Model file for the job. Use its own axes, mm. Face numbers are marked on the shaded views. A direction names the side the tool comes from. Give positions to 0.01 mm unless a question says otherwise; leave off trailing zeros. Write each loop counter-clockwise with the first axis right and the second up, starting at its lowest first coordinate (ties: lowest second). Pieces come first, ordered by that corner, then holes. Notation, with made-up numbers: (60.25, -6) - (105.25, -6) arc R18 ccw to (105.25, 2) - close; hole circle Ø2 at (-24.5, 42). An arc over 180 degrees is marked (long way). One line per item, written item: value. Start each with the question number.
(1) Mould opens along Z. For the marked faces 1, 2 and 3 say: pulls with the +Z half, pulls with the -Z half, needs draft (parallel to the pull), parting line crosses it, or undercut.
(2) Cut at A-A, the plane y = 0. List the corners of the cut face in (x, z).
(3) 3-axis set-ups, long thin cutter, end or side, ignore diameter. For the marked faces 4, 5, 6 and 7: which of +Z, -Z, +X, -X, +Y, -Y reach the whole face in a straight line?
(4) Drop flat-ended pins along their axis: P1, Ø3, axis at y = 14, z = 39.5, coming from the -X side; P2, Ø3, axis at x = 13.5, z = -13, coming from the +Y side; P3, Ø17, axis at x = 0, y = 0, coming from the +Z side; P4, Ø12, axis at x = 0, y = 0, coming from the -Z side. Give the stop position or say it passes through.
(5) Cut at D-D, the plane y = 17. List the corners of the cut face in (x, z).
(6) Cut at C-C, the plane z = 19.5. List the corners of the cut face in (x, y).
(7) Probe L1, parallel to X at y = 0, z = -16; L2, parallel to Y at x = 0, z = 22.5; L3, parallel to Y at x = 0, z = 35.5. List the from-to ranges inside material, lowest first.
(8) Cut at B-B, the plane x = 0. List the corners of the cut face in (y, z).
from build123d import *

# Parameters (mm, degrees)
F0_W          = 60
F0_H          = 50
F1_DEPTH      = 25
F1_DEPTH_BACK = 25
F4_R          = 7.5
F5_DEPTH      = 75.001
F6_R          = 12.5
F7_DEPTH      = 35
F7_DEPTH_BACK = 35


with BuildPart() as f1:
    # F0 (on Top) → F1 (new body, two sides)
    with BuildSketch(Plane.XY) as f1_sk:
        Rectangle(F0_W, F0_H)
    extrude(amount=F1_DEPTH)
    extrude(f1_sk.sketch, amount=-F1_DEPTH_BACK)

    # F2 (on Front) → F3 (revolve)
    with BuildSketch(Plane.XZ):
        Polygon((-15, 40), (-15, 25), (0, 25), (0, 50), (-25, 50), (-25, 40), align=None)
    revolve(axis=Axis((0, 0, 37.5), (0, 0, -1)))

    # F4 (on face) → F5 (cut, through all)
    with BuildSketch(Plane.XY.offset(50)):
        Circle(F4_R)
    extrude(amount=-F5_DEPTH, mode=Mode.SUBTRACT)

    # F6 (on Front) → F7 (join, two sides)
    with BuildSketch(Plane.XZ) as f7_sk:
        Circle(F6_R)
    extrude(amount=F7_DEPTH)
    extrude(f7_sk.sketch, amount=-F7_DEPTH_BACK)


solid = f1.part
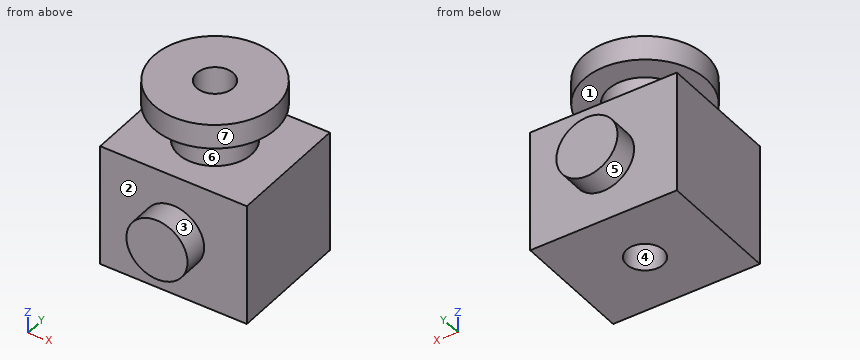
Answers follow:
1. face 1: undercut
1. face 2: needs draft
1. face 3: parting line crosses it
2. outline: (-30, -25) - (-7.5, -25) - (-7.5, -10) arc R12.5 ccw to (7.5, -10) - (7.5, -25) - (30, -25) - (30, 25) - (15, 25) - (15, 40) - (25, 40) - (25, 50) - (7.5, 50) - (7.5, 10) arc R12.5 ccw to (-7.5, 10) - (-7.5, 50) - (-25, 50) - (-25, 40) - (-15, 40) - (-15, 25) - (-30, 25) - close
3. face 4: -Z
3. face 5: +Y
3. face 6: none
3. face 7: +Z
4. P1: stops at x = -21.6
4. P2: stops at y = 25
4. P3: stops at z = 50
4. P4: stops at z = -12.5
5. outline: (-30, -25) - (30, -25) - (30, 25) - (-30, 25) - close; (-18.33, 40) - (18.33, 40) - (18.33, 50) - (-18.33, 50) - close
6. outline: (-30, -25) - (30, -25) - (30, 25) - (-30, 25) - close; hole circle Ø15 at (0, 0)
7. L1: x = -30 to -7.5, 7.5 to 30
7. L2: y = -25 to -7.5, 7.5 to 25
7. L3: y = -15 to -7.5, 7.5 to 15
8. outline: (-35, -12.5) - (-25, -12.5) - (-25, -25) - (-7.5, -25) - (-7.5, -12.5) - (7.5, -12.5) - (7.5, -25) - (25, -25) - (25, -12.5) - (35, -12.5) - (35, 12.5) - (25, 12.5) - (25, 25) - (15, 25) - (15, 40) - (25, 40) - (25, 50) - (7.5, 50) - (7.5, 12.5) - (-7.5, 12.5) - (-7.5, 50) - (-25, 50) - (-25, 40) - (-15, 40) - (-15, 25) - (-25, 25) - (-25, 12.5) - (-35, 12.5) - close
